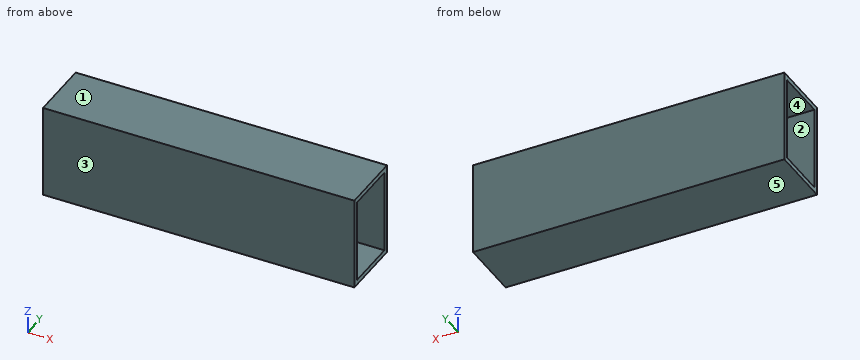
from build123d import *

# Parameters (mm, degrees)
F0_W     = 254
F0_H     = 50.8
F1_DEPTH = 76.2
F2_T     = -3.9878
F3_DEPTH = 3.9888


with BuildPart() as f1:
    # F0 (on Top) → F1 (new body)
    with BuildSketch(Plane.XY):
        with Locations((127, 25.4)):
            Rectangle(F0_W, F0_H)
    extrude(amount=F1_DEPTH)

    # F2
    f2_openings = [f1.faces().sort_by_distance(p)[0] for p in [
        (254, 25.4, 38.1),
    ]]
    offset(amount=F2_T, openings=f2_openings)

    # F3 (cut, through all): a face of the model
    f3_faces = [f1.faces().sort_by_distance(p)[0] for p in [
        (3.9878, 25.4, 38.1),
    ]]
    extrude(f3_faces, amount=-F3_DEPTH, mode=Mode.SUBTRACT)


solid = f1.part
CAD build for the part. Positions are in the model's coordinates, mm. Face numbers are marked on the shaded views. A direction names the side the tool comes from. Round coordinates to 2 decimals unless told otherwise and drop trailing zeros. Order: outer loops, then holes, each group sorted by start corner. A loop starts at its lowest first (then second) coordinate and runs counter-clockwise, first axis right, second up. Notation, with made-up numbers: (29.5, -24.75) - (44.5, -24.75) arc R37 ccw to (44.5, 13.25) - close; hole circle Ø1 at (66, -34). An arc over 180 degrees is marked (long way). Return JSON: item names as keys, results as strings.
(1) Pin check, flat tip, straight feed: pin 1 Ø21.5 at (x, y) = (114.5, 22) entering from -Z. Stop position of the tip, or through.
Answer key:
{"pin 1": "stops at z = 0"}
(2) Pull direction Z, two halves, no side cores. Call the marked faces 1, 2 and 3: +Z half, -Z half, draft (parallel to the pull), parting line (faces both ways), or undercut.
Answer key:
{"face 1": "+Z half", "face 2": "undercut", "face 3": "draft"}
(3) Cut at C-C (x = 186.5). Give the cut face in (y, z).
Answer key:
{"outline": "(0, 0) - (50.8, 0) - (50.8, 76.2) - (0, 76.2) - close; hole (3.99, 3.99) - (46.81, 3.99) - (46.81, 72.21) - (3.99, 72.21) - close"}
(4) Cut at B-B (z = 18.5). Give the cut face in (x, y).
Answer key:
{"outline": "(0, 0) - (254, 0) - (254, 3.99) - (0, 3.99) - close; (0, 46.81) - (254, 46.81) - (254, 50.8) - (0, 50.8) - close"}
(5) Cut at A-A (y = 35). Give the cut face in (x, z), then the cut area to 3 significant figures.
Answer key:
{"outline": "(0, 0) - (254, 0) - (254, 3.99) - (0, 3.99) - close; (0, 72.21) - (254, 72.21) - (254, 76.2) - (0, 76.2) - close", "area": "2,030 mm^2"}
(6) Wall check: probe 1 along Z at (x, y) = (18.5, 34); probe 2 along Y at (x, z) = (175.5, 14). Give the ranges that are in metal, low to high. Write a range as from..to.
Answer key:
{"probe 1": "z = 0..3.99, 72.21..76.2", "probe 2": "y = 0..3.99, 46.81..50.8"}
(7) Tool access for the marked faces 4 and 5: list every direction of +Z, -Z, +X, -X, +Y, -Y with a clear straight run to the whole face (end or side of a thin tool).
Answer key:
{"face 4": "+X, -X", "face 5": "-Z, +X, -X, +Y, -Y"}
